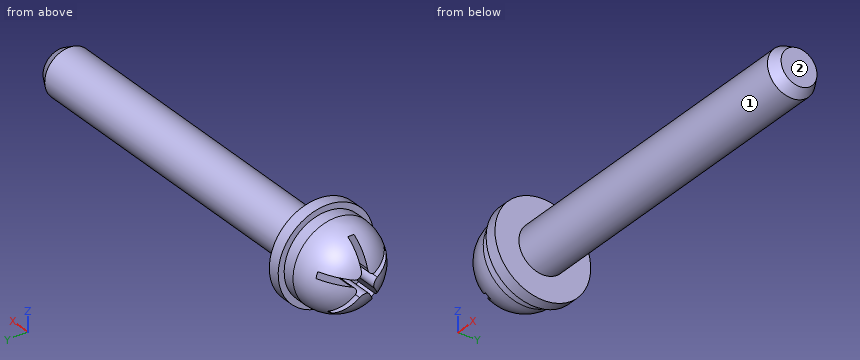
```python
from build123d import *

# Parameters (mm, degrees)
SKETCH2_R               = 2
BOSS_EXTRUDE1_DEPTH     = 28.866025404
CUT_EXTRUDE1_REACH      = 33.38
CUT_EXTRUDE1_END_RADIUS = 3.5
CHAMFER1_SIZE           = 0.5
CHAMFER1_SIZE2          = 0.866025404
FILLET1_R               = 0.5


with BuildPart() as part:
    # Sketch1 → Revolve1 (revolve)
    with BuildSketch(Plane(origin=(0, 0, 0), x_dir=(-1, 0, 0), z_dir=(0, 0, -1)), mode=Mode.PRIVATE) as revolve1_sk:
        with BuildLine():
            Line((14, 4), (14, 0))
            Line((14, 0), (19.5, 0))
            ThreePointArc((19.5, 0), (18.474873734, 2.474873734), (16, 3.5))
            Line((16, 3.5), (15, 3.5))
            Line((15, 3.5), (15, 4))
            Line((15, 4), (14, 4))
        make_face()
    revolve(revolve1_sk.sketch.rotate(Axis((-14, 0, 0), (-1, 0, 0)), 270), axis=Axis((-14, 0, 0), (-1, 0, 0)))

    # Sketch2 → Boss-Extrude1 (add)
    with BuildSketch(Plane(origin=(-14, 0, 0), x_dir=(0, 0, -1), z_dir=(1, 0, 0))):
        Circle(SKETCH2_R)
    extrude(amount=BOSS_EXTRUDE1_DEPTH)

    # Cut-Extrude1: up to this sphere (the profile starts inside it)
    cut_extrude1_end = Location((-16, 0, 0)) * Sphere(CUT_EXTRUDE1_END_RADIUS, mode=Mode.PRIVATE)
    # Sketch3 → Cut-Extrude1 (cut, up to the surface)
    with BuildSketch(Plane(origin=(-16, 0, 0), x_dir=(0, 0, -1), z_dir=(1, 0, 0)), mode=Mode.PRIVATE) as cut_extrude1_sk1:
        with BuildLine():
            Line((2.267866263, 1.963869297), (0.134474286, 0.413869297))
            Line((0.134474286, 0.413869297), (-0.680408938, 2.921821979))
            ThreePointArc((-0.680408938, 2.921821979), (-0.927050983, 2.853169549), (-1.166941475, 2.763737975))
            Line((-1.166941475, 2.763737975), (-0.352058252, 0.255785292))
            Line((-0.352058252, 0.255785292), (-2.989075758, 0.255785292))
            ThreePointArc((-2.989075758, 0.255785292), (-3, 0), (-2.989075758, -0.255785292))
            Line((-2.989075758, -0.255785292), (-0.352058252, -0.255785292))
            Line((-0.352058252, -0.255785292), (-1.166941475, -2.763737975))
            ThreePointArc((-1.166941475, -2.763737975), (-0.927050983, -2.853169549), (-0.680408938, -2.921821979))
            Line((-0.680408938, -2.921821979), (0.134474286, -0.413869297))
            Line((0.134474286, -0.413869297), (2.267866263, -1.963869297))
            ThreePointArc((2.267866263, -1.963869297), (2.427050983, -1.763355757), (2.568559908, -1.55))
            Line((2.568559908, -1.55), (0.435167931, 0))
            Line((0.435167931, 0), (2.568559908, 1.55))
            ThreePointArc((2.568559908, 1.55), (2.427050983, 1.763355757), (2.267866263, 1.963869297))
        make_face()
    cut_extrude1_tool1 = extrude(cut_extrude1_sk1.sketch, amount=-CUT_EXTRUDE1_REACH, mode=Mode.PRIVATE) & cut_extrude1_end
    add(cut_extrude1_tool1.solids().sort_by_distance((-16, 0, 0))[0], mode=Mode.SUBTRACT)

    # Chamfer1
    chamfer1_edges = [part.edges().sort_by_distance(p)[0] for p in [
        (14.866025404, 0, 2),
    ]]
    chamfer1_side = [part.faces().sort_by_distance(p)[0] for p in [
        (14.866025404, 0, 0),
    ]]
    chamfer(chamfer1_edges, length=CHAMFER1_SIZE, length2=CHAMFER1_SIZE2, reference=chamfer1_side[0])

    # Fillet1
    # the kernel refuses this fillet: 0.5 mm, written as the material it takes off along each edge
    with BuildSketch(Plane(origin=(-16, 0, -0.435167931), x_dir=(0, -0.5877852522924764, -0.8090169943749451), z_dir=(-1, 0, 0)), Plane(origin=(-16, -0.413869297, -0.134474286), x_dir=(0, -0.9510565162951523, 0.3090169943749514), z_dir=(-1, 0, 0)), Plane(origin=(-16, -0.255785292, 0.352058252), x_dir=(0, 0, 1), z_dir=(-1, 0, 0)), Plane(origin=(-16, 0.255785292, 0.352058252), x_dir=(0, 0.9510565162951548, 0.3090169943749436), z_dir=(-1, 0, 0)), Plane(origin=(-16, 0.413869297, -0.134474286), x_dir=(0, 0.5877852522924701, -0.8090169943749497), z_dir=(-1, 0, 0))) as fillet1_piece_1:
        with BuildLine():
            CenterArc((FILLET1_R * 1.37638192047, -FILLET1_R), FILLET1_R, 90, 108)
            Line((FILLET1_R * 0.425325404176, -FILLET1_R * 1.30901699437), (0, 0))
            Line((0, 0), (FILLET1_R * 1.37638192047, 0))
        make_face()
    extrude(amount=5.193319014, mode=Mode.SUBTRACT)


solid = part.part
```
Part model, mm, in its own coordinate system. Face numbers are marked on the shaded views. A direction names the side the tool comes from. Round coordinates to 2 decimals unless told otherwise and drop trailing zeros. Order: outer loops, then holes, each group sorted by start corner. A loop starts at its lowest first (then second) coordinate and runs counter-clockwise, first axis right, second up. Notation, with made-up numbers: M 86.5,0.25 L 135.5,0.25 A22 cw 135.5,32.25 Z; hole C 43.25,1 d9. An arc over 180 degrees is marked long. Put each result on its own line as item: value. Start each with the question number.
1. Slice it at A-A on x = -3. List the corners of the cut face in (y, z).
2. Tool access for the marked faces 1 and 2: list every direction of +Z, -Z, +X, -X, +Y, -Y with a clear straight run to the whole face (end or side of a thin tool).
3. Drop flat-ended pins along their axis: pin 1 (2 mm diameter, centred on x = -18.5, z = 2, fed in from -Y); pin 2 (2.5 mm diameter, centred on y = 1.5, z = 1.5, fed in from +X); pin 3 (0.6 mm diameter, centred on x = -17, z = 2.5, fed in from +Y); pin 4 (1.5 mm diameter, centred on y = -2.5, z = -1, fed in from +X). Give the stop position or say it passes through.
4. Drill centre lines: probe 1 along X at (y, z) = (0, -0.5); probe 2 along Z at (x, y) = (-16.5, 2.25); probe 3 along Z at (x, y) = (-17, -0.5). Where is each one in solid material? Low to high. Write a range as [from, to].
Findings:
1. outline: C 0,0 d4
2. face 1: +X
2. face 2: +Z, -Z, +X, +Y, -Y
3. pin 1: y = -2.72
3. pin 2: x = 14.87
3. pin 3: y = 2.55
3. pin 4: x = 14.1
4. probe 1: [-16, 14.87]
4. probe 2: [-2.63, 0.46], [1, 2.63]
4. probe 3: [-3.32, -1.12], [0.61, 3.32]
